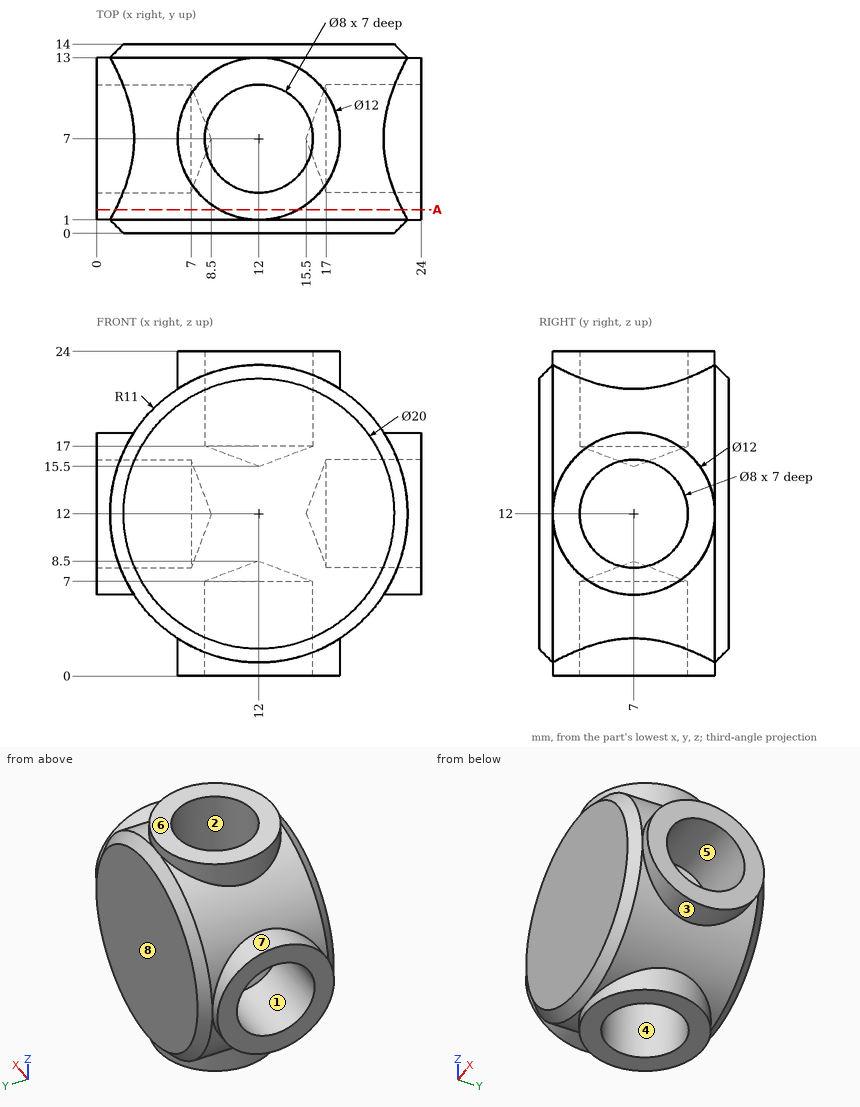
Geometry: see drawing. Coordinates: mm, zero at the bounding-box minimum. A direction names the side the tool comes from. Round coordinates to 2 decimals unless told otherwise and drop trailing zeros. Write each loop counter-clockwise with the first axis right and the second up, starting at its lowest first coordinate (ties: lowest second). Pieces come first, ordered by that corner, then holes. Notation, with made-up numbers: M 6,-31 L 54,-31 A18 cw 54,2 Z; hole C 75,87.25 d2. An arc over 180 degrees is marked long. Answer in a Markdown table with one row per item. Add a question column.
(1) Cut plane A-A, the plane y = 1.75. Return the cut outline in (x, z), then the cut area to 3 significant figures.
(2) Ray query, L1, parallel to Z at x = 21.5, y = 7; L2, parallel to Z at x = 21, y = 7. Return the intervals inside material, ascending.
(3) Draft query along Z for the marked faces 5, 6, 7 and 8. Return one class per face: pulls with the +Z half, pulls with the -Z half, needs draft (parallel to the pull), parting line crosses it, or undercut.
(4) Contact query for flat-ended pins moving along their axis: pin 1 (1 mm diameter, centred on x = 13.5, y = 8, fed in from +Z); pin 2 (5 mm diameter, centred on x = 3.5, y = 10, fed in from +Z); pin 3 (7 mm diameter, centred on y = 7, z = 12, fed in from -X). Output: stop coordinate, or through.
(5) Reachability of the marked faces 1, 2, 3 and 4 from +Z, -Z, +X, -X, +Y, -Y: full face, straight path, thin tool, end or side. Return the list, or none.
Established:
| question | item | result |
|---|---|---|
| 1 | outline | M 0,9.1 L 1.39,9.1 A11 ccw 9.1,1.39 L 9.1,0 L 14.9,0 L 14.9,1.39 A11 ccw 22.61,9.1 L 24,9.1 L 24,14.9 L 22.61,14.9 A11 ccw 14.9,22.61 L 14.9,24 L 9.1,24 L 9.1,22.61 A11 ccw 1.39,14.9 L 0,14.9 Z |
| 1 | area | 406 mm² |
| 2 | L1 | 6 to 8, 16 to 18 |
| 2 | L2 | 5.68 to 8, 16 to 18.32 |
| 3 | face 5 | undercut |
| 3 | face 6 | pulls with the +Z half |
| 3 | face 7 | parting line crosses it |
| 3 | face 8 | needs draft |
| 4 | pin 1 | z = 16.36 |
| 4 | pin 2 | z = 21.22 |
| 4 | pin 3 | x = 7.19 |
| 5 | face 1 | -X |
| 5 | face 2 | +Z |
| 5 | face 3 | +X |
| 5 | face 4 | -Z |
